Work out the finished part from the listing and answer in its coordinate system (mm). Coordinates: 2 decimals unless noted, no trailing zeros. Loops run counter-clockwise (first coordinate to the right, second up) from the corner with the lowest first, then second, coordinate; pieces in that order, holes last. Notation, with made-up numbers: (24, -19) -> (44, -19) arc R25 ccw to (44, 17) -> close; hole circle Ø7 at (-22.5, 64.5). An arc over 180 degrees is marked (long way). Use a Markdown table: item, result. Add a question column.
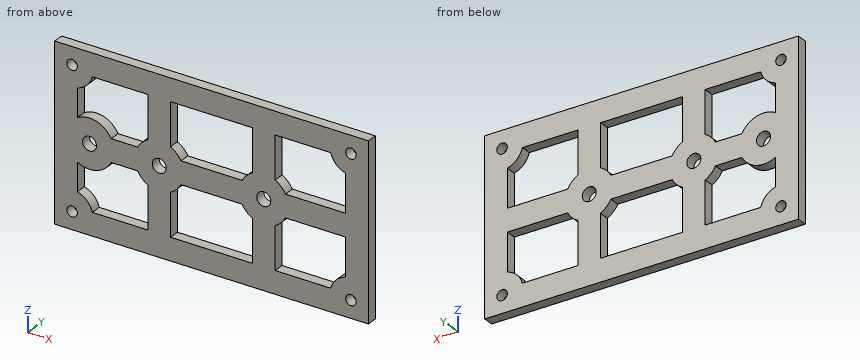
```python
from build123d import *

# Parameters (mm, degrees)
SKETCH1_W           = 90
SKETCH1_H           = 50
BOSS_EXTRUDE1_DEPTH = 3
SKETCH3_R           = 2
CUT_EXTRUDE2_DEPTH  = 10
SKETCH2_R           = 1.5
CUT_EXTRUDE3_DEPTH  = 10


with BuildPart() as part:
    # Sketch1 → Boss-Extrude1 (new body)
    with BuildSketch(Plane(origin=(0, 0, 0), x_dir=(1, 0, 0), z_dir=(0, 1, 0))):
        Rectangle(SKETCH1_W, SKETCH1_H)
    extrude(amount=BOSS_EXTRUDE1_DEPTH)

    # Sketch3 → Cut-Extrude2 (cut)
    with BuildSketch(Plane(origin=(0, 3, 0), x_dir=(1, 0, 0), z_dir=(0, 1, 0))):
        with Locations(Location((-35, 0, 0), (0, 0, 270))):
            Circle(SKETCH3_R)
        with Locations(Location((-15, 0, 0), (0, 0, 270))):
            Circle(SKETCH3_R)
        with Locations(Location((15, 0, 0), (0, 0, 270))):
            Circle(SKETCH3_R)
    extrude(amount=-CUT_EXTRUDE2_DEPTH, mode=Mode.SUBTRACT)

    # Sketch2 → Cut-Extrude3 (cut)
    with BuildSketch(Plane(origin=(0, 3, 0), x_dir=(1, 0, 0), z_dir=(0, 1, 0))):
        with Locations(Location((-40, -20, 0), (0, 0, 270))):
            Circle(SKETCH2_R)
        with Locations(Location((40, -20, 0), (0, 0, 270))):
            Circle(SKETCH2_R)
        with Locations(Location((40, 20, 0), (0, 0, 270))):
            Circle(SKETCH2_R)
        with Locations(Location((-40, 20, 0), (0, 0, 270))):
            Circle(SKETCH2_R)
        with BuildLine():
            Line((38.5, -14.190524981), (38.5, -6.062177826))
            Line((38.5, -6.062177826), (38.5, -3.25))
            Line((38.5, -3.25), (28.800201616, -3.25))
            Line((28.800201616, -3.25), (21.199798384, -3.25))
            ThreePointArc((21.199798384, -3.25), (19.949747468, -4.949747468), (18.25, -6.199798384))
            Line((18.25, -6.199798384), (18.25, -18.5))
            Line((18.25, -18.5), (34.190524981, -18.5))
            ThreePointArc((34.190524981, -18.5), (35.757359313, -15.757359313), (38.5, -14.190524981))
        make_face()
        with BuildLine():
            Line((-34.190524981, -18.5), (-18.25, -18.5))
            Line((-18.25, -18.5), (-18.25, -6.199798384))
            ThreePointArc((-18.25, -6.199798384), (-19.949747468, -4.949747468), (-21.199798384, -3.25))
            Line((-21.199798384, -3.25), (-28.800201616, -3.25))
            ThreePointArc((-28.800201616, -3.25), (-33.05081713, -6.723145554), (-38.5, -6.062177826))
            Line((-38.5, -6.062177826), (-38.5, -14.190524981))
            ThreePointArc((-38.5, -14.190524981), (-35.757359313, -15.757359313), (-34.190524981, -18.5))
        make_face()
        with BuildLine():
            Line((38.5, 14.190524981), (38.5, 6.062177826))
            Line((38.5, 6.062177826), (38.5, 3.25))
            Line((38.5, 3.25), (28.800201616, 3.25))
            Line((28.800201616, 3.25), (21.199798384, 3.25))
            ThreePointArc((21.199798384, 3.25), (19.949747468, 4.949747468), (18.25, 6.199798384))
            Line((18.25, 6.199798384), (18.25, 18.5))
            Line((18.25, 18.5), (34.190524981, 18.5))
            ThreePointArc((34.190524981, 18.5), (35.757359313, 15.757359313), (38.5, 14.190524981))
        make_face()
        with BuildLine():
            Line((-38.5, 14.190524981), (-38.5, 6.062177826))
            ThreePointArc((-38.5, 6.062177826), (-33.05081713, 6.723145554), (-28.800201616, 3.25))
            Line((-28.800201616, 3.25), (-21.199798384, 3.25))
            ThreePointArc((-21.199798384, 3.25), (-19.949747468, 4.949747468), (-18.25, 6.199798384))
            Line((-18.25, 6.199798384), (-18.25, 18.5))
            Line((-18.25, 18.5), (-34.190524981, 18.5))
            ThreePointArc((-34.190524981, 18.5), (-35.757359313, 15.757359313), (-38.5, 14.190524981))
        make_face()
        with BuildLine():
            Line((-11.75, 18.5), (11.75, 18.5))
            Line((11.75, 18.5), (11.75, 6.199798384))
            ThreePointArc((11.75, 6.199798384), (10.050252532, 4.949747468), (8.800201616, 3.25))
            Line((8.800201616, 3.25), (-8.800201616, 3.25))
            ThreePointArc((-8.800201616, 3.25), (-10.050252532, 4.949747468), (-11.75, 6.199798384))
            Line((-11.75, 6.199798384), (-11.75, 18.5))
        make_face()
        with BuildLine():
            Line((-11.75, -18.5), (11.75, -18.5))
            Line((11.75, -18.5), (11.75, -6.199798384))
            ThreePointArc((11.75, -6.199798384), (10.050252532, -4.949747468), (8.800201616, -3.25))
            Line((8.800201616, -3.25), (-8.800201616, -3.25))
            ThreePointArc((-8.800201616, -3.25), (-10.050252532, -4.949747468), (-11.75, -6.199798384))
            Line((-11.75, -6.199798384), (-11.75, -18.5))
        make_face()
    extrude(amount=-CUT_EXTRUDE3_DEPTH, mode=Mode.SUBTRACT)


solid = part.part
```
Item 1: Find the intervals of material crossed by probe 1 along X at (y, z) = (1.45, 20); probe 2 along Z at (x, y) = (8.5, 2.1), in increasing order.
Item 2: Section D-D (z = -10) is taken. Determine the outline of the cut face in (x, y).
Item 3: Section B-B (z = 20) is taken. Determine the outline of the cut face in (x, y).
Item 4: Section A-A (x = 15) is taken. Determine the outline of the cut face in (y, z).
Item 5: Given pin 1 (3.5 mm diameter, centred on x = 40, z = 20, fed in from +Y), flat-ended and moving along its own axis, determine where the tip first touches the part or whether it passes through.
Item 6: Section C-C (x = 40) is taken. Determine the outline of the cut face in (y, z).
Output:
| question | item | result |
|---|---|---|
| 1 | probe 1 | x = -45 to -41.5, -38.5 to 38.5, 41.5 to 45 |
| 1 | probe 2 | z = -25 to -18.5, -3.25 to 3.25, 18.5 to 25 |
| 2 | outline | (-45, 0) -> (-38.5, 0) -> (-38.5, 3) -> (-45, 3) -> close; (-18.25, 0) -> (-11.75, 0) -> (-11.75, 3) -> (-18.25, 3) -> close; (11.75, 0) -> (18.25, 0) -> (18.25, 3) -> (11.75, 3) -> close; (38.5, 0) -> (45, 0) -> (45, 3) -> (38.5, 3) -> close |
| 3 | outline | (-45, 0) -> (-41.5, 0) -> (-41.5, 3) -> (-45, 3) -> close; (-38.5, 0) -> (38.5, 0) -> (38.5, 3) -> (-38.5, 3) -> close; (41.5, 0) -> (45, 0) -> (45, 3) -> (41.5, 3) -> close |
| 4 | outline | (0, -25) -> (3, -25) -> (3, -2) -> (0, -2) -> close; (0, 2) -> (3, 2) -> (3, 25) -> (0, 25) -> close |
| 5 | pin 1 | stops at y = 3 |
| 6 | outline | (0, -25) -> (3, -25) -> (3, -21.5) -> (0, -21.5) -> close; (0, -18.5) -> (3, -18.5) -> (3, 18.5) -> (0, 18.5) -> close; (0, 21.5) -> (3, 21.5) -> (3, 25) -> (0, 25) -> close |
